The listing builds one solid part. Answer for the finished solid, in the listing's coordinates (mm). Face numbers are marked on the shaded views. Coordinates: 2 decimals unless noted, no trailing zeros. Loops run counter-clockwise (first coordinate to the right, second up) from the corner with the lowest first, then second, coordinate; pieces in that order, holes last. Notation, with made-up numbers: (74.25, 18.5) - (91.25, 18.5) arc R28 ccw to (91.25, 57.5) - close; hole circle Ø2 at (-24.75, -20.5). An arc over 180 degrees is marked (long way). Put each result on its own line as item: value.
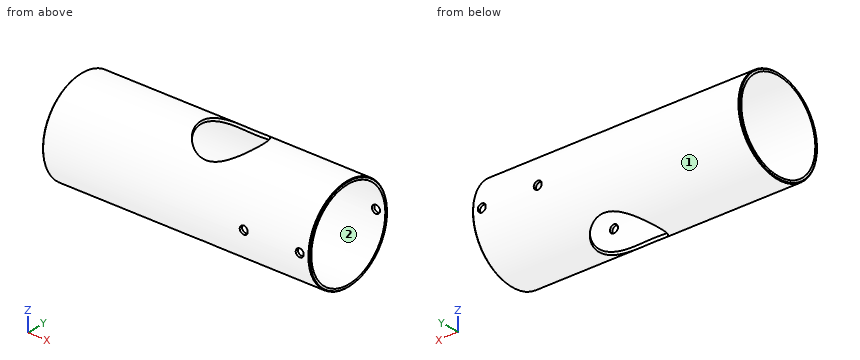
Solid Edge part; units mm, degrees
sketch "Sketch1" plane through (0, 0, 0) normal (0, -1, 0) x (1, 0, 0)
  line L0 (-100, 33) -> (100, 33)
  line L1 (100, 33) -> (100, 35)
  line L2 (100, 35) -> (-100, 35)
  line L3 (-100, 35) -> (-100, 33)
  dimension "D1" = 100
  dimension "D2" = 100
revolve "RevolvedProtrusion1" add sketch "Sketch1" angle 360 about axis through (-60, 0, 0) along (1, 0, 0)
chamfer "pipe_chamfers" distance 0.5 angle 45 2 edges at (100, 0, -35) (-100, 0, -35)
sketch "Sketch2" plane through (0, 0, 0) normal (0, 0, 1) x (1, 0, 0)
  circle A0 centre (12, 0) radius 22.5
extrude "pipe_cutout" cut sketch "Sketch2" along normal mid plane 100
sketch "Sketch3" plane through (0, 0, 0) normal (0, -1, 0) x (1, 0, 0)
  circle A0 centre (93, 0) radius 3
  circle A1 centre (51, 0) radius 3
extrude "pin_cutouts_Profile_Plane1" cut sketch "Sketch3" along normal mid plane 100
properties material "Aluminum, 1060"
1) For a pull along Y with two mould halves and no side action, classify the marked faces 1 and 2 as pulls with the +Y half, pulls with the -Y half, needs draft (parallel to the pull), parting line crosses it, or undercut.
Found:
face 1: parting line crosses it
face 2: undercut
2) The part is cut by section A-A (z = 0). Give the vertices of the cut face in (x, y), and give its area (4 significant figures).
Found:
outline: (-100, -34.5) - (-99.5, -35) - (48, -35) - (48, -33) - (-100, -33) - close; (-100, 33) - (48, 33) - (48, 35) - (-99.5, 35) - (-100, 34.5) - close; (54, -35) - (90, -35) - (90, -33) - (54, -33) - close; (54, 33) - (90, 33) - (90, 35) - (54, 35) - close; (96, -35) - (99.5, -35) - (100, -34.5) - (100, -33) - (96, -33) - close; (96, 33) - (100, 33) - (100, 34.5) - (99.5, 35) - (96, 35) - close
area: 751.5 mm^2
3) The part is cut by section C-C (x = 51). Give the vertices of the cut face in (y, z).
Found:
outline: (-34.87, -3) arc R35 ccw to (34.87, -3) - (32.86, -3) arc R33 cw to (-32.86, -3) - close; (-34.87, 3) - (-32.86, 3) arc R33 cw to (32.86, 3) - (34.87, 3) arc R35 ccw to start
4) Straight lines are drawn through the part: L1, parallel to X at y = -34.4, z = 0; L2, parallel to Z at x = -36, y = 0. For each, find the intervals that lie inside material, in ascending order. Write a range as [from, to].
Found:
L1: x = [-100, 48], [54, 90], [96, 100]
L2: z = [-35, -33], [33, 35]
5) The part is cut by section B-B (y = 0). Give the vertices of the cut face in (x, z).
Found:
outline: (-100, -34.5) - (-99.5, -35) - (-10.5, -35) - (-10.5, -33) - (-100, -33) - close; (-100, 33) - (-10.5, 33) - (-10.5, 35) - (-99.5, 35) - (-100, 34.5) - close; (34.5, -35) - (99.5, -35) - (100, -34.5) - (100, -33) - (34.5, -33) - close; (34.5, 33) - (100, 33) - (100, 34.5) - (99.5, 35) - (34.5, 35) - close
6) Each of these flat-tipped pins is pushed along its axis until it touches: pin 1 (4 mm diameter, centred on x = -70, y = 4.5, fed in from +Z); pin 2 (12 mm diameter, centred on x = -70, z = 7.5, fed in from +Y); pin 3 (3 mm diameter, centred on x = -48.5, z = -20, fed in from +Y). Where does it stop, or does it pass through?
Found:
pin 1: stops at z = 34.91
pin 2: stops at y = 34.97
pin 3: stops at y = 29.71
7) The part is cut by section D-D (x = -77). Give the vertices of the cut face in (y, z), and give its area (3 significant figures).
Found:
outline: circle Ø70 at (0, 0); hole circle Ø66 at (0, 0)
area: 427 mm^2
